from build123d import *

# Parameters (mm, degrees)
SKETCH2_R           = 3.175
SKETCH2_R_2         = 2
SKETCH2_R_3         = 1.5875
SKETCH2_R_4         = 1.999999991
BOSS_EXTRUDE1_DEPTH = 5.588


with BuildPart() as part:
    # Sketch2 → Boss-Extrude1 (new body)
    with BuildSketch(Plane(origin=(0, 0, 0), x_dir=(1, 0, 0), z_dir=(0, 1, 0))):
        with BuildLine():
            Line((15.15555913, -28.018449791), (13.238676936, -27.713033224))
            ThreePointArc((13.238676936, -27.713033224), (11.241051513, -26.538356195), (10.573787778, -24.319092227))
            Line((10.573787778, -24.319092227), (12.5603, 0))
            ThreePointArc((12.5603, 0), (0.603657177, 12.545785512), (-12.502275592, 1.2059192))
            Line((-12.502275592, 1.2059192), (-16.498266045, -40.222207921))
            ThreePointArc((-16.498266045, -40.222207921), (-16.507064815, -40.344000039), (-16.51, -40.466074291))
            Line((-16.51, -40.466074291), (-16.51, -221.328861788))
            ThreePointArc((-16.51, -221.328861788), (-12.970187584, -225.680718913), (-7.988667969, -223.101301399))
            Line((-7.988667969, -223.101301399), (16.979901226, -165.677523619))
            ThreePointArc((16.979901226, -165.677523619), (17.216065593, -164.934164738), (17.295902343, -164.158289667))
            Line((17.295902343, -164.158289667), (17.295902343, -30.526810701))
            ThreePointArc((17.295902343, -30.526810701), (16.688093876, -28.878103365), (15.15555913, -28.018449791))
        make_face()
        with Locations(Location((0, 0, 0), (0, 0, 270))):
            Circle(SKETCH2_R, mode=Mode.SUBTRACT)
        with Locations(Location((-11.43, -219.075, 0), (0, 0, 270))):
            Circle(SKETCH2_R_2, mode=Mode.SUBTRACT)
        with Locations(Location((-11.43, -212.725, 0), (0, 0, 270))):
            Circle(SKETCH2_R_2, mode=Mode.SUBTRACT)
        with Locations(Location((-11.43, -206.375, 0), (0, 0, 270))):
            Circle(SKETCH2_R_2, mode=Mode.SUBTRACT)
        with Locations(Location((-11.43, -200.025, 0), (0, 0, 270))):
            Circle(SKETCH2_R_2, mode=Mode.SUBTRACT)
        with Locations(Location((-12.7, -82.55, 0), (0, 0, 270))):
            Circle(SKETCH2_R_3, mode=Mode.SUBTRACT)
        with Locations(Location((13.485902343, -38.1, 0), (0, 0, 270))):
            Circle(SKETCH2_R_4, mode=Mode.SUBTRACT)
        with Locations(Location((13.485902343, -162.410770806, 0), (0, 0, 270))):
            Circle(SKETCH2_R_2, mode=Mode.SUBTRACT)
        with BuildLine():
            Line((10.438542905, -167.981776143), (-0.534170778, -193.217289931))
            ThreePointArc((-0.534170778, -193.217289931), (-2.234040931, -194.665234867), (-4.420389569, -194.211381682))
            Line((-4.420389569, -194.211381682), (-11.716886202, -188.551043102))
            ThreePointArc((-11.716886202, -188.551043102), (-12.441018517, -187.661516081), (-12.7, -186.544128716))
            Line((-12.7, -186.544128716), (-12.7, -149.615408258))
            ThreePointArc((-12.7, -149.615408258), (-11.988693683, -148.474898999), (-10.651556899, -148.611951065))
            Line((-10.651556899, -148.611951065), (7.135902343, -162.410770806))
            ThreePointArc((7.135902343, -162.410770806), (8.023611961, -165.648962244), (10.438542905, -167.981776143))
        make_face(mode=Mode.SUBTRACT)
        with BuildLine():
            Line((-7.44734835, -76.074408803), (7.575478058, -45.053638233))
            ThreePointArc((7.575478058, -45.053638233), (8.043996088, -44.531101035), (8.718495671, -44.337182032))
            Line((8.718495671, -44.337182032), (10.945902343, -44.337182032))
            ThreePointArc((10.945902343, -44.337182032), (11.843927955, -44.70915642), (12.215902343, -45.607182032))
            Line((12.215902343, -45.607182032), (12.215902343, -119.492817968))
            ThreePointArc((12.215902343, -119.492817968), (11.264685124, -120.722158254), (9.835937715, -120.109971535))
            Line((9.835937715, -120.109971535), (-7.44734835, -89.025591197))
            ThreePointArc((-7.44734835, -89.025591197), (-5.976040897, -82.55), (-7.44734835, -76.074408803))
        make_face(mode=Mode.SUBTRACT)
        with BuildLine():
            Line((-12.431479451, -37.743315662), (-9.755434212, -9.99962016))
            ThreePointArc((-9.755434212, -9.99962016), (-2.756273581, -13.695395429), (5.127655889, -12.99492382))
            Line((5.127655889, -12.99492382), (3.069264048, -38.19397392))
            ThreePointArc((3.069264048, -38.19397392), (2.259083254, -39.854914801), (0.537695935, -40.527182032))
            Line((0.537695935, -40.527182032), (-9.903213406, -40.527182032))
            ThreePointArc((-9.903213406, -40.527182032), (-11.783508673, -39.694838236), (-12.431479451, -37.743315662))
        make_face(mode=Mode.SUBTRACT)
        with BuildLine():
            Line((1.663048834, -44.337182032), (-10.16, -44.337182032))
            ThreePointArc((-10.16, -44.337182032), (-11.956051224, -45.081130808), (-12.7, -46.877182032))
            Line((-12.7, -46.877182032), (-12.7, -74.6125))
            ThreePointArc((-12.7, -74.6125), (-11.873503915, -74.655646925), (-11.055993219, -74.784618621))
            Line((-11.055993219, -74.784618621), (2.806066447, -46.160725831))
            ThreePointArc((2.806066447, -46.160725831), (2.739129831, -44.932682449), (1.663048834, -44.337182032))
        make_face(mode=Mode.SUBTRACT)
        with BuildLine():
            Line((8.923603828, -154.049487576), (-10.733772403, -138.80005889))
            ThreePointArc((-10.733772403, -138.80005889), (-12.182037035, -137.021004847), (-12.7, -134.786230117))
            Line((-12.7, -134.786230117), (-12.7, -90.4875))
            ThreePointArc((-12.7, -90.4875), (-11.888769677, -90.445936399), (-11.086035141, -90.321680879))
            Line((-11.086035141, -90.321680879), (11.575760855, -131.079432803))
            ThreePointArc((11.575760855, -131.079432803), (12.053263487, -132.272915946), (12.215902343, -133.548047069))
            Line((12.215902343, -133.548047069), (12.215902343, -152.970817152))
            ThreePointArc((12.215902343, -152.970817152), (10.520298026, -153.359206519), (8.923603828, -154.049487576))
        make_face(mode=Mode.SUBTRACT)
    extrude(amount=BOSS_EXTRUDE1_DEPTH)


solid = part.part
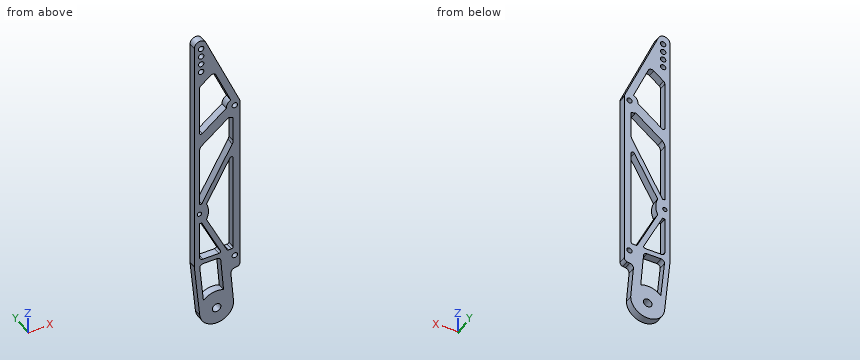
Geometry: final body of the model. Coordinates: model frame, mm. Give positions to 0.01 mm unless a question says otherwise; leave off trailing zeros. Write each loop counter-clockwise with the first axis right and the second up, starting at its lowest first coordinate (ties: lowest second). Pieces come first, ordered by that corner, then holes. Notation, with made-up numbers: (-3, 61) -> (22, 61) arc R17 ccw to (22, 68) -> close; hole circle Ø5 at (62.5, 52). An arc over 180 degrees is marked (long way). Answer as a JSON object with one key per item and string values.
1. Cut plane A-A on z = 87. Output: boundary loops of the cut face in (x, y), and give its area (3 significant figures).
Ans:
{"outline": "(-16.51, 0) -> (-6.65, 0) -> (-6.65, 5.59) -> (-16.51, 5.59) -> close; (12.22, 0) -> (17.3, 0) -> (17.3, 5.59) -> (12.22, 5.59) -> close", "area": "83.5 mm^2"}
2. Ray query, probe 1 along Z at (x, y) = (9, 4.8); probe 2 along Z at (x, y) = (13.5, 2.75); probe 3 along X at (y, z) = (4.4, 59.5). Return the intervals inside material, ascending. Write a range as from..to.
Ans:
{"probe 1": "z = -8.76..44.34, 118.61..126.45, 154.01..166.91, 171.29..184.03", "probe 2": "z = 27.75..36.1, 40.1..160.41, 164.41..173.68", "probe 3": "x = -16.51..-12.7, -3.65..0.58, 12.22..17.3"}
3. Cut plane C-C on z = 18. Output: boundary loops of the cut face in (x, y), and give its area (3 significant figures).
Ans:
{"outline": "(-14.35, 0) -> (-10.53, 0) -> (-10.53, 5.59) -> (-14.35, 5.59) -> close; (4.72, 0) -> (11.09, 0) -> (11.09, 5.59) -> (4.72, 5.59) -> close", "area": "57.0 mm^2"}
4. Cut plane B-B on y = 1.65. Count the separate pieces of the cut face and the enclosed holes in it, and give its area (3 significant figures).
Ans:
{"separate pieces": "1", "enclosed holes": "13", "area": "3,440 mm^2"}
5. Contact query for flat-ended pins moving along their axis: pin 1 (3 mm diameter, centred on x = 13.5, y = 3.5, fed in from +Z); pin 2 (1.7 mm diameter, centred on x = -6.5, y = 4, fed in from +Z); pin 3 (1.8 mm diameter, centred on x = 10, y = 4, fed in from +Z). Output: stop coordinate, or through.
Ans:
{"pin 1": "stops at z = 177.13", "pin 2": "stops at z = 221.63", "pin 3": "stops at z = 183.8"}
